Input: dimensioned drawing with shaded views. Units: mm. Origin: part minimum x, y, z. Give positions to 0.01 mm unless a question says otherwise; leave off trailing zeros. Write each loop counter-clockwise with the first axis right and the second up, starting at its lowest first coordinate (ties: lowest second). Pieces come first, ordered by that corner, then holes.
Q1. Section C-C (x = 101). Return the cut outline in (y, z), plus the area to 3 significant figures.
Q2. Line query: line 1 (X direction, y = 364.5, z = 179); line 2 (X direction, y = 248.5, z = 55.5). Output: solid intervals per line, ascending.
Q3. Section D-D (z = 83.5). Return the cut outline in (x, y), plus the area to 3 significant figures.
Q4. Mould query, pull axis Y, two halves, no side actions, for the marked faces 1, 2, 3 and 4. Classes: +Y half, -Y half, draft (parallel to the pull), parting line (faces both ways), or undercut.
Q5. Section A-A (y = 87.5). Return the cut outline in (x, z), plus the area to 3 significant figures.
Q6. Section B-B (z = 119). Return the cut outline in (x, y) (1 decimal), plus the area to 3 significant figures.
Q7. Pin query (flat end, axial travel): pin 1 Ø10 at (y, z) = (248, 58) entering from -X. Return the tip coordinate at first contact, or that it passes through.
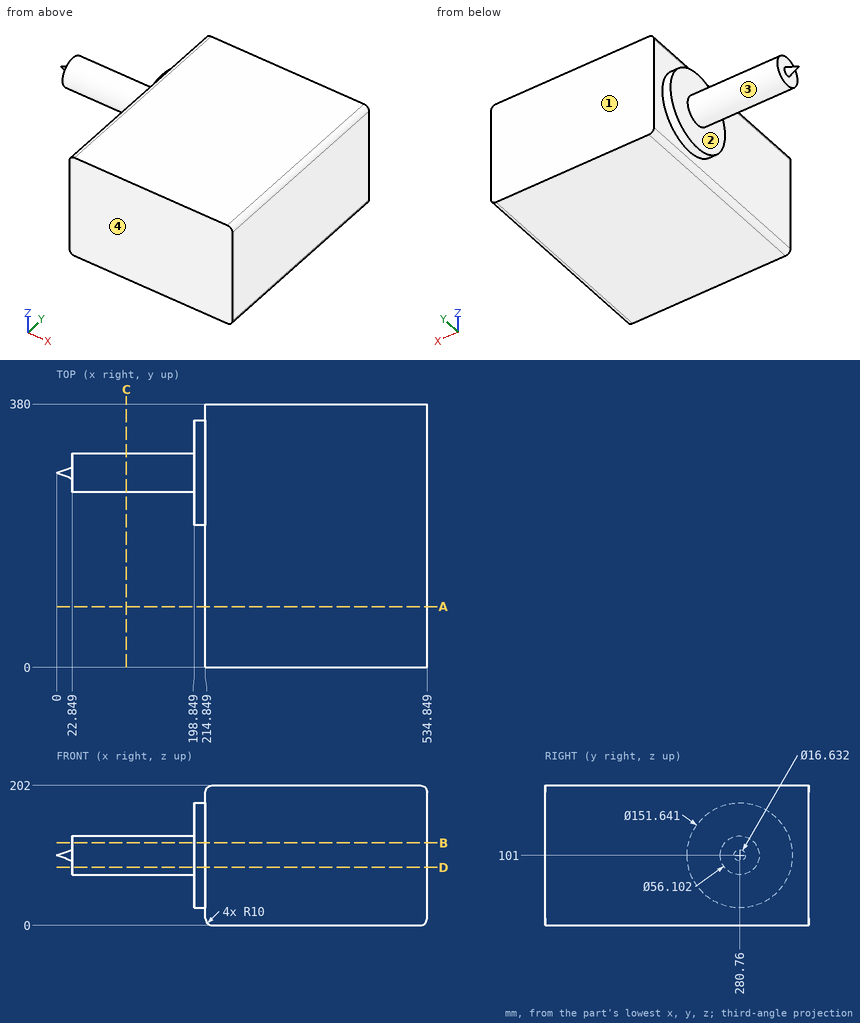
Computed:
1. outline: circle Ø56.1 at (280.76, 101)
1. area: 2,470 mm2
2. line 1: x = 214.85 to 534.85
2. line 2: x = 198.85 to 534.85
3. outline: (22.85, 258.84) - (198.85, 258.84) - (198.85, 206.99) - (214.85, 206.99) - (214.85, 0) - (534.85, 0) - (534.85, 380) - (214.85, 380) - (214.85, 354.53) - (198.85, 354.53) - (198.85, 302.68) - (22.85, 302.68) - close
3. area: 132,000 mm2
4. face 1: +Y half
4. face 2: draft
4. face 3: parting line
4. face 4: -Y half
5. outline: (214.85, 10) arc R10 ccw to (224.85, 0) - (524.85, 0) arc R10 ccw to (534.85, 10) - (534.85, 192) arc R10 ccw to (524.85, 202) - (224.85, 202) arc R10 ccw to (214.85, 192) - close
5. area: 64,600 mm2
6. outline: (22.8, 259.2) - (198.8, 259.2) - (198.8, 207.1) - (214.8, 207.1) - (214.8, 0) - (534.8, 0) - (534.8, 380) - (214.8, 380) - (214.8, 354.4) - (198.8, 354.4) - (198.8, 302.3) - (22.8, 302.3) - close
6. area: 132,000 mm2
7. pin 1: stops at x = 198.85
